Could you check a few things on this model? Use its own coordinates, in mm. Coordinates: 2 decimals unless noted, no trailing zeros. Loops run counter-clockwise (first coordinate to the right, second up) from the corner with the lowest first, then second, coordinate; pieces in that order, holes last. Notation, with made-up numbers: (21, 32) -> (64, 32) arc R12 cw to (64, 38) -> close; hole circle Ø6 at (-33.5, 23). An arc over 180 degrees is marked (long way). One line per question, with ' | ' between items.
```python
from build123d import *

# Parameters (mm, degrees)
SKETCH1_W            = 95
SKETCH1_H            = 75
SKETCH1_W_2          = 24.25
SKETCH1_H_2          = 11
BOSS_EXTRUDE1_DEPTH  = 4.5
SKETCH2_R            = 1.45
SCREWHOLES_DEPTH     = 61.685665523
SKETCH4_R            = 1.45
SKETCH4_W            = 9.8
SKETCH4_H            = 4.4
CUT_EXTRUDE3_DEPTH   = 61.685665523
SKETCH5_R            = 1.45
SKETCH5_W            = 4.4
SKETCH5_H            = 9.8
CUT_EXTRUDE4_DEPTH   = 61.685665523
SKETCH9_R            = 4
SKETCH9_R_2          = 1.45
BOSS_EXTRUDE3_DEPTH  = 4.5
SKETCH10_W           = 10
SKETCH10_H           = 75
CUT_EXTRUDE5_DEPTH   = 62.623859016
BOSS_EXTRUDE4_DEPTH  = 4.5
SKETCH12_R           = 1.45
FANBRACESCREWS_DEPTH = 55.290883213
SKETCH13_W           = 42
SKETCH13_H           = 14
CUT_EXTRUDE7_DEPTH   = 55.290883213
SKETCH15_R           = 1.45
BELTCLIPSCREWS_DEPTH = 55.290883213


with BuildPart() as part:
    # Sketch1 → Boss-Extrude1 (new body)
    with BuildSketch(Plane.XY):
        Rectangle(SKETCH1_W, SKETCH1_H)
        with Locations((-22.125, 22.5)):
            Rectangle(SKETCH1_W_2, SKETCH1_H_2, mode=Mode.SUBTRACT)
        with Locations((22.125, 22.5)):
            Rectangle(SKETCH1_W_2, SKETCH1_H_2, mode=Mode.SUBTRACT)
        with Locations((22.125, -22.5)):
            Rectangle(SKETCH1_W_2, SKETCH1_H_2, mode=Mode.SUBTRACT)
        with Locations((-22.125, -22.5)):
            Rectangle(SKETCH1_W_2, SKETCH1_H_2, mode=Mode.SUBTRACT)
    extrude(amount=BOSS_EXTRUDE1_DEPTH)

    # Sketch2 → screwHoles (cut, through all)
    with BuildSketch(Plane.XY.offset(4.5)):
        with Locations((-30, 35)):
            Circle(SKETCH2_R)
        with Locations(Location((30, 35, 0), (0, 0, 180))):
            Circle(SKETCH2_R)
        with Locations((40, 0)):
            Circle(SKETCH2_R)
        with Locations(Location((-40, 0, 0), (0, 0, 180))):
            Circle(SKETCH2_R)
        with Locations((0, 35)):
            Circle(SKETCH2_R)
    extrude(amount=-SCREWHOLES_DEPTH, mode=Mode.SUBTRACT)

    # Sketch4 → Cut-Extrude3 (cut, through all)
    with BuildSketch(Plane.XY.offset(4.5)):
        Circle(SKETCH4_R)
        with Locations((-25, 0)):
            Rectangle(SKETCH4_W, SKETCH4_H)
        with Locations((25, 0)):
            Rectangle(SKETCH4_W, SKETCH4_H)
    extrude(amount=-CUT_EXTRUDE3_DEPTH, mode=Mode.SUBTRACT)

    # Sketch5 → Cut-Extrude4 (cut, through all)
    with BuildSketch(Plane.XY.offset(4.5)):
        with Locations((33, -31.75)):
            Circle(SKETCH5_R)
        with Locations(Location((-33, -31.75, 0), (0, 0, 180))):
            Circle(SKETCH5_R)
        with Locations((33, -9.75)):
            Rectangle(SKETCH5_W, SKETCH5_H)
        with Locations((-33, -9.75)):
            Rectangle(SKETCH5_W, SKETCH5_H)
    extrude(amount=-CUT_EXTRUDE4_DEPTH, mode=Mode.SUBTRACT)

    # Sketch9 → Boss-Extrude3 (add, through all)
    # profile 1 of 2: a face of its own
    with BuildSketch(Plane.XY.offset(4.5)):
        with Locations((-30, 35)):
            Circle(SKETCH9_R)
        with Locations((-30, 35)):
            Circle(SKETCH9_R_2, mode=Mode.SUBTRACT)
    # profile 2 of 2: a face of its own
    with BuildSketch(Plane.XY.offset(4.5)):
        with Locations((30, 35)):
            Circle(SKETCH9_R)
        with Locations(Location((30, 35, 0), (0, 0, 180))):
            Circle(SKETCH9_R_2, mode=Mode.SUBTRACT)
    extrude(amount=-BOSS_EXTRUDE3_DEPTH)

    # Sketch10 → Cut-Extrude5 (cut, through all)
    with BuildSketch(Plane.XY.offset(4.5)):
        with Locations((-42.5, 0)):
            Rectangle(SKETCH10_W, SKETCH10_H)
        with Locations((42.5, 0)):
            Rectangle(SKETCH10_W, SKETCH10_H)
    extrude(amount=-CUT_EXTRUDE5_DEPTH, mode=Mode.SUBTRACT)

    # Sketch11 → Boss-Extrude4 (add, through all)
    with BuildSketch(Plane.XY.offset(4.5)):
        Polygon((-30, 39), (30, 39), (26.877501001, 37.5), (-26.877501001, 37.5), align=None)
    extrude(amount=-BOSS_EXTRUDE4_DEPTH)

    # Sketch12 → FanBraceScrews (cut, through all)
    with BuildSketch(Plane.XY.offset(4.5)):
        with Locations((-16, -8.25)):
            Circle(SKETCH12_R)
        with Locations(Location((16, -8.25, 0), (0, 0, 180))):
            Circle(SKETCH12_R)
    extrude(amount=-FANBRACESCREWS_DEPTH, mode=Mode.SUBTRACT)

    # Sketch13 → Cut-Extrude7 (cut, through all)
    with BuildSketch(Plane.XY.offset(4.5)):
        with Locations((0, -37.5)):
            Rectangle(SKETCH13_W, SKETCH13_H)
    extrude(amount=-CUT_EXTRUDE7_DEPTH, mode=Mode.SUBTRACT)

    # Sketch15 → BeltClipScrews (cut, through all)
    with BuildSketch(Plane.XY.offset(4.5)):
        with Locations((-25, 5.25)):
            Circle(SKETCH15_R)
        with Locations((-25, -6.75)):
            Circle(SKETCH15_R)
        with Locations(Location((25, -6.75, 0), (0, 0, 180))):
            Circle(SKETCH15_R)
        with Locations(Location((25, 5.25, 0), (0, 0, 180))):
            Circle(SKETCH15_R)
    extrude(amount=-BELTCLIPSCREWS_DEPTH, mode=Mode.SUBTRACT)


solid = part.part
```
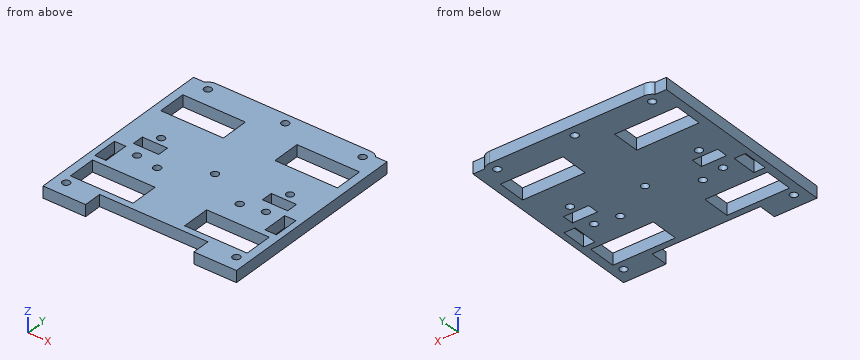
Q1. Imagine slicing it at D-D on x = 25. Write out the boundary of the cut face in (y, z), plus the area to 3 significant figures.
Values follow:
outline: (-37.5, 0) -> (-28, 0) -> (-28, 4.5) -> (-37.5, 4.5) -> close; (-17, 0) -> (-8.2, 0) -> (-8.2, 4.5) -> (-17, 4.5) -> close; (-5.3, 0) -> (-2.2, 0) -> (-2.2, 4.5) -> (-5.3, 4.5) -> close; (2.2, 0) -> (3.8, 0) -> (3.8, 4.5) -> (2.2, 4.5) -> close; (6.7, 0) -> (17, 0) -> (17, 4.5) -> (6.7, 4.5) -> close; (28, 0) -> (39, 0) -> (39, 4.5) -> (28, 4.5) -> close | area: 199 mm2
Q2. Imagine slicing it at B-B on y = -31.75. Write out the boundary of the cut face in (x, z).
Values follow:
outline: (-37.5, 0) -> (-34.45, 0) -> (-34.45, 4.5) -> (-37.5, 4.5) -> close; (-31.55, 0) -> (-21, 0) -> (-21, 4.5) -> (-31.55, 4.5) -> close; (21, 0) -> (31.55, 0) -> (31.55, 4.5) -> (21, 4.5) -> close; (34.45, 0) -> (37.5, 0) -> (37.5, 4.5) -> (34.45, 4.5) -> close
Q3. Imagine slicing it at C-C on y = 5.25. Write out the boundary of the cut face in (x, z), plus the area to 3 significant figures.
Values follow:
outline: (-37.5, 0) -> (-26.45, 0) -> (-26.45, 4.5) -> (-37.5, 4.5) -> close; (-23.55, 0) -> (23.55, 0) -> (23.55, 4.5) -> (-23.55, 4.5) -> close; (26.45, 0) -> (37.5, 0) -> (37.5, 4.5) -> (26.45, 4.5) -> close | area: 311 mm2
Q4. Please list where these lines run through material, in increasing order: L1, parallel to X at y = -11.5, z = 0.75; L2, parallel to X at y = -20, z = 0.5; L3, parallel to Y at x = -30, z = 2.1. Write a range as [from, to].
Values follow:
L1: x = [-37.5, -35.2], [-30.8, 30.8], [35.2, 37.5] | L2: x = [-37.5, -34.25], [-10, 10], [34.25, 37.5] | L3: y = [-37.5, -28], [-17, 17], [28, 33.55], [36.45, 39]
Q5. For pin 1 (2 mm diameter, centred on x = -35, z = 1.5, fed in from +Y); pin 2 (2 mm diameter, centred on x = 33.5, z = 3, fed in from +Y), each with a flat end and sliding along its axis, tell me the tip position at first contact or that it passes through.
Values follow:
pin 1: stops at y = 37.5 | pin 2: stops at y = 38.12
Q6. Imagine slicing it at A-A on x = 16. Write out the boundary of the cut face in (y, z).
Values follow:
outline: (-30.5, 0) -> (-28, 0) -> (-28, 4.5) -> (-30.5, 4.5) -> close; (-17, 0) -> (-9.7, 0) -> (-9.7, 4.5) -> (-17, 4.5) -> close; (-6.8, 0) -> (17, 0) -> (17, 4.5) -> (-6.8, 4.5) -> close; (28, 0) -> (39, 0) -> (39, 4.5) -> (28, 4.5) -> close
